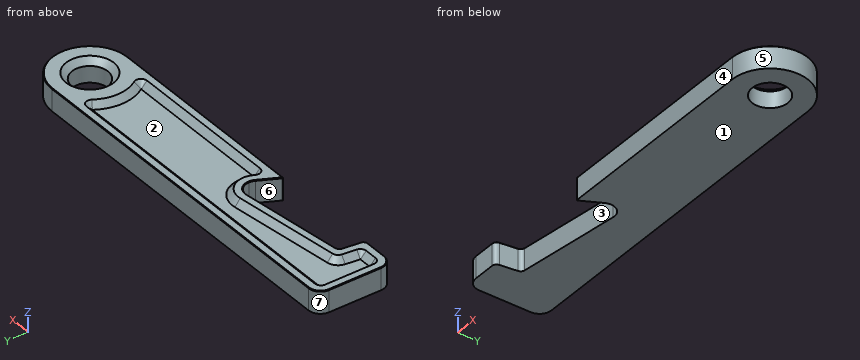
from build123d import *

# Parameters (mm, degrees)
F0_R     = 6
F1_DEPTH = 7.5
F3_DEPTH = 2
F4_SIZE  = 1.99999
F5_SIZE  = 2
F6_SIZE  = 0.2


# Not quite as in the source:
# - a fillet or chamfer is up to 0.001 mm smaller than in the source, because OpenCascade refuses the exact size


with BuildPart() as f1:
    # F0 (on Top) → F1 (new body)
    with BuildSketch(Plane.XY):
        with BuildLine():
            Line((0, 12.7), (-116.65, 12.7))
            ThreePointArc((-116.65, 12.7), (-119.4784271247, 11.5284271247), (-120.65, 8.7))
            Line((-120.65, 8.7), (-120.65, -8.7))
            ThreePointArc((-120.65, -8.7), (-119.4784271247, -11.5284271247), (-116.65, -12.7))
            Line((-116.65, -12.7), (-109.2756163486, -12.7))
            ThreePointArc((-109.2756163486, -12.7), (-108.2823049478, -12.323980632), (-107.7869993139, -11.3844432814))
            Line((-107.7869993139, -11.3844432814), (-107.0773577752, -5.6570214144))
            ThreePointArc((-107.0773577752, -5.6570214144), (-106.6508978642, -4.7823035915), (-105.77738814, -4.3533745914))
            Line((-105.77738814, -4.3533745914), (-71.4370597318, 0))
            ThreePointArc((-71.4370597318, 0), (-68.2894054117, -0.967220541), (-66.934, -3.9682402783))
            ThreePointArc((-66.934, -3.9682402783), (-67.0466854589, -4.910994572), (-67.3783928291, -5.8006315156))
            Line((-67.3783928291, -5.8006315156), (-70.7461413924, -12.3354755477))
            ThreePointArc((-70.7461413924, -12.3354755477), (-70.7373768459, -12.5801324074), (-70.5239159442, -12.7))
            Line((-70.5239159442, -12.7), (0, -12.7))
            ThreePointArc((0, -12.7), (12.7, 0), (0, 12.7))
        make_face()
        Circle(F0_R, mode=Mode.SUBTRACT)
    extrude(amount=F1_DEPTH)

    # F2 (on face) → F3 (cut)
    with BuildSketch(Plane.XY.offset(7.5)):
        with BuildLine():
            ThreePointArc((-10.5404901245, -7.0843537415), (-12.7, 0), (-10.5404901245, 7.0843537415))
            ThreePointArc((-10.5404901245, 7.0843537415), (-10.4352904965, 9.1404008409), (-12.2004098292, 10.2))
            Line((-12.2004098292, 10.2), (-116.15, 10.2))
            ThreePointArc((-116.15, 10.2), (-117.5642135624, 9.6142135624), (-118.15, 8.2))
            Line((-118.15, 8.2), (-118.15, -8.2))
            ThreePointArc((-118.15, -8.2), (-117.5642135624, -9.6142135624), (-116.15, -10.2))
            Line((-116.15, -10.2), (-111.9268490457, -10.2))
            ThreePointArc((-111.9268490457, -10.2), (-110.6024338446, -9.6986408426), (-109.9420263328, -8.4459243752))
            Line((-109.9420263328, -8.4459243752), (-109.3672424661, -3.8069207262))
            ThreePointArc((-109.3672424661, -3.8069207262), (-108.7986292513, -2.6406302958), (-107.6339496191, -2.0687249623))
            Line((-107.6339496191, -2.0687249623), (-71.7514720642, 2.4801501739))
            ThreePointArc((-71.7514720642, 2.4801501739), (-68.3008484478, 1.9745295223), (-65.6082269333, -0.2418289696))
            ThreePointArc((-65.6082269333, -0.2418289696), (-64.4404924053, -3.6777938671), (-65.2968047441, -7.2042918302))
            ThreePointArc((-65.2968047441, -7.2042918302), (-65.2930945463, -9.2021436175), (-63.5622831269, -10.2))
            Line((-63.5622831269, -10.2), (-12.2004098292, -10.2))
            ThreePointArc((-12.2004098292, -10.2), (-10.4352904965, -9.1404008409), (-10.5404901245, -7.0843537415))
        make_face()
    extrude(amount=-F3_DEPTH, mode=Mode.SUBTRACT)

    # F4 (size 2 in the source; OpenCascade refuses exactly that, so slightly less here)
    f4_edges = [f1.edges().sort_by_distance(p)[0] for p in [
        (-12.7, 0, 5.5),
        (-10.43529, 9.140401, 5.5),
        (-64.175205, 10.2, 5.5),
        (-117.564214, 9.614214, 5.5),
        (-118.15, 0, 5.5),
        (-117.564214, -9.614214, 5.5),
        (-114.038425, -10.2, 5.5),
        (-110.602434, -9.698641, 5.5),
        (-109.654634, -6.126423, 5.5),
        (-108.798629, -2.64063, 5.5),
        (-89.692711, 0.205713, 5.5),
        (-65.525254, -0.363318, 5.5),
        (-65.293095, -9.202144, 5.5),
        (-37.881346, -10.2, 5.5),
        (-10.43529, -9.140401, 5.5),
    ]]
    chamfer(f4_edges, length=F4_SIZE)

    # F5
    f5_edges = [f1.edges().sort_by_distance(p)[0] for p in [
        (-6, 0, 7.5),
    ]]
    chamfer(f5_edges, length=F5_SIZE)

    # F6
    f6_edges = [f1.edges().sort_by_distance(p)[0] for p in [
        (-58.325, 12.7, 7.5),
    ]]
    chamfer(f6_edges, length=F6_SIZE)


solid = f1.part
Geometry: final body of the model. Coordinates: model frame, mm. Face numbers are marked on the shaded views. A direction names the side the tool comes from. Round coordinates to 2 decimals unless told otherwise and drop trailing zeros. Order: outer loops, then holes, each group sorted by start corner. A loop starts at its lowest first (then second) coordinate and runs counter-clockwise, first axis right, second up. Notation, with made-up numbers: (62, -6) -> (100, -6) arc R11 ccw to (100, 7) -> close; hole circle Ø1 at (64.5, 62.25). An arc over 180 degrees is marked (long way). Put each result on its own line as item: value. Start each with the question number.
Q1. Pull-direction query (X, two-part tool) for the marked faces 4, 5, 6 and 7; classes: +X half, -X half, draft (parallel to the pull), parting line (faces both ways), or undercut.
Q2. First-contact query: pin 1 (1.5 mm diameter, centred on x = -75.5, z = 6, fed in from -Y); pin 2 (5 mm diameter, centred on x = -52.5, y = 1.5, fed in from +Z). Flat tips, straight axial feed; report the tip coordinate or a pass-through.
Q3. Section A-A on z = 3.5. Return the cut outline in (x, y), and give its area (3 significant figures).
Q4. Reachability of the marked faces 1, 2 and 3 from +Z, -Z, +X, -X, +Y, -Y: full face, straight path, thin tool, end or side. Return the list, or none.
Q5. Line query: probe 1 along X at (y, z) = (5.25, 7); probe 2 along X at (y, z) = (4.5, 6.5); probe 3 along Z at (x, y) = (-19, 7.5). Output: solid intervals per line, ascending.
Ans:
1. face 4: draft
1. face 5: +X half
1. face 6: undercut
1. face 7: -X half
2. pin 1: stops at y = -0.61
2. pin 2: stops at z = 5.5
3. outline: (-120.65, -8.7) arc R4 ccw to (-116.65, -12.7) -> (-109.28, -12.7) arc R1.5 ccw to (-107.79, -11.38) -> (-107.08, -5.66) arc R1.5 cw to (-105.78, -4.35) -> (-71.44, 0) arc R4 cw to (-67.38, -5.8) -> (-70.75, -12.34) arc R0.25 ccw to (-70.52, -12.7) -> (0, -12.7) arc R12.7 ccw to (0, 12.7) -> (-116.65, 12.7) arc R4 ccw to (-120.65, 8.7) -> close; hole circle Ø12 at (0, 0)
3. area: 2,780 mm2
4. face 1: -Z, +X, -X, +Y, -Y
4. face 2: +Z
4. face 3: +Z, -Z, -Y
5. probe 1: x = -120.65 to -117.65, -12.11 to -5.36, 5.36 to 11.56
5. probe 2: x = -120.65 to -117.15, -12.94 to -5.36, 5.36 to 11.88
5. probe 3: z = 0 to 5.5
